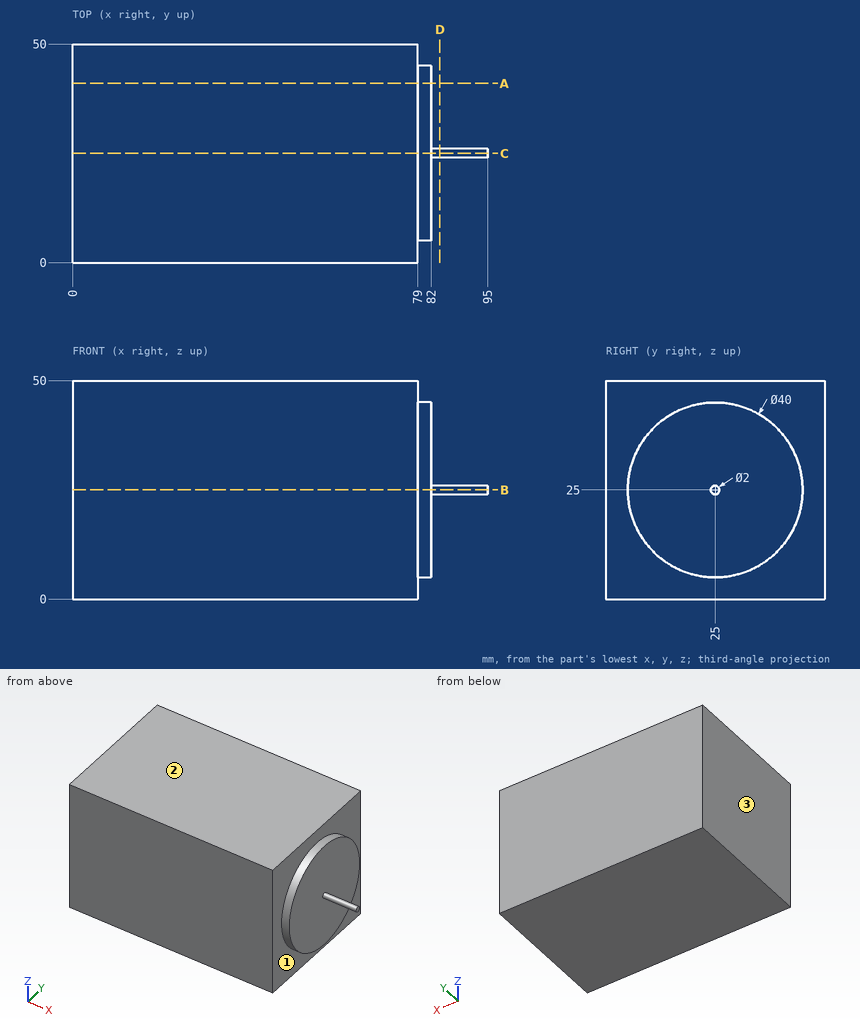
For this review, use the dimensioned drawing (mm, ordinates from the lowest corner) and the shaded views. Give positions to 0.01 mm unless a question says otherwise; leave off trailing zeros. Write each loop counter-clockwise with the first axis right and the second up, starting at its lowest first coordinate (ties: lowest second). Pieces come first, ordered by that corner, then holes.
(1) Consider section A-A, the plane y = 41. Give the boundary of the cut face in (x, z), and give its area (3 significant figures).
(2) Consider section D-D, the plane x = 84. Give the boundary of the cut face in (y, z), and give its area (3 significant figures).
(3) Consider section B-B, the plane z = 25. Give the boundary of the cut face in (x, y), and give its area (3 significant figures).
(4) To check wall thickness, follow L1, parallel to X at y = 17, z = 17.5; L2, parallel to X at y = 31, z = 5.5. State the ranges of each line that lie inside material, in increasing order.
(5) The part is to be moulded in two halves that separate along X. For the marked faces 1, 2 and 3, say which applies: released by +X, released by -X, zero draft, split by the parting line, or undercut.
(6) For P1, Ø6, axis at x = 84, z = 12.5, coming from the -Y side; P2, Ø1, axis at y = 44.5, z = 35, coming from the +X side, all flat-tipped, find the tip position at first contact; note any pin that passes through.
Returned:
1. outline: (0, 0) - (79, 0) - (79, 13) - (82, 13) - (82, 37) - (79, 37) - (79, 50) - (0, 50) - close
1. area: 4,020 mm2
2. outline: circle Ø2 at (25, 25)
2. area: 3.14 mm2
3. outline: (0, 0) - (79, 0) - (79, 5) - (82, 5) - (82, 24) - (95, 24) - (95, 26) - (82, 26) - (82, 45) - (79, 45) - (79, 50) - (0, 50) - close
3. area: 4,100 mm2
4. L1: x = 0 to 82
4. L2: x = 0 to 79
5. face 1: released by +X
5. face 2: zero draft
5. face 3: released by -X
6. P1: stops at y = 7.83
6. P2: stops at x = 79
